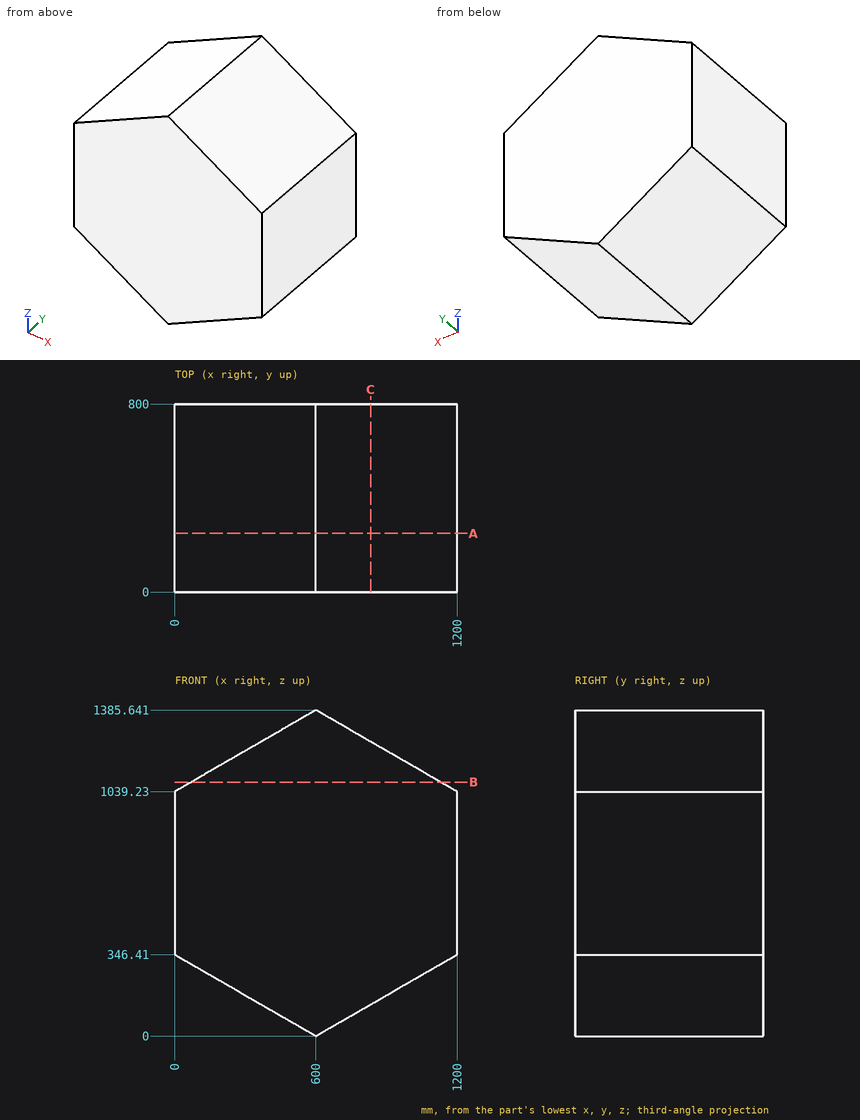
Answer from the drawing. Dimensions are ordinates in mm from the lowest x, y and z of the part. Give positions to 0.01 mm unless a question says otherwise; leave off trailing zeros. Order: outer loops, then holes, each group sorted by start corner. A loop starts at its lowest first (then second) coordinate and runs counter-clockwise, first axis right, second up. Notation, with made-up numbers: (-18, -2) -> (0, -2) arc R21 ccw to (0, 9) -> close; hole circle Ø5 at (-27, -9). An arc over 180 degrees is marked (long way). One line per item, written item: value. Start each with the question number.
(1) The part is cut by section C-C (x = 832.5). Determine the outline of the cut face in (y, z), and give its area (3 significant figures).
(2) The part is cut by section A-A (y = 250). Determine the outline of the cut face in (x, z).
(3) Straight lines are drawn through the part: L1, parallel to Z at x = 885, y = 507.5 (1 decimal); L2, parallel to Z at x = 310, y = 357; L3, parallel to X at y = 217.5, z = 1274 (1 decimal). For each, find the intervals that lie inside material, in ascending order.
(4) Flat-ended cylindrical pins translate along their axes: P1, Ø1.5, axis at x = 922.5, y = 175, coming from the +Z side; P2, Ø1, axis at x = 906.5, y = 87.5, coming from the -Z side; P3, Ø2, axis at y = 234, z = 285, coming from the +X side (1 decimal). Find the tip coordinate at first contact, or state that the pin passes through.
(5) The part is cut by section B-B (z = 1080). Determine the outline of the cut face in (x, y) (1 decimal).
Taken from the geometry:
1. outline: (0, 134.23) -> (800, 134.23) -> (800, 1251.41) -> (0, 1251.41) -> close
1. area: 894,000 mm^2
2. outline: (0, 346.41) -> (600, 0) -> (1200, 346.41) -> (1200, 1039.23) -> (600, 1385.64) -> (0, 1039.23) -> close
3. L1: 164.5 to 1221.1
3. L2: 167.43 to 1218.21
3. L3: 406.6 to 793.4
4. P1: z = 1199.88
4. P2: z = 176.67
4. P3: x = 1095.4
5. outline: (70.6, 0) -> (1129.4, 0) -> (1129.4, 800) -> (70.6, 800) -> close
